Source: three-view drawing plus pictorial views. Frame: mm from the lowest corner of the part. Give positions to 0.01 mm unless a question says otherwise; leave off trailing zeros. Loops run counter-clockwise (first coordinate to the right, second up) from the corner with the lowest first, then second, coordinate; pieces in that order, holes last. Notation, with made-up numbers: M 28.5,68.25 L 32.5,68.25 A19 cw 32.5,85.25 Z; hole C 76.25,85.5 d7. An arc over 180 degrees is marked long. One line per item, written item: value. Start each with the question number.
(1) Ray query, line 1 along Y through (x, z) = (39.95, 2.3); line 2 along Y through (x, z) = (27.5, 2.1); line 3 along X through (y, z) = (59, 1.25). Return the intervals inside material, ascending. Write a range as from..to.
(2) Section B-B on x = 27.5. Output: boundary loops of the cut face in (y, z).
(3) Pin query (flat end, axial travel): P1, Ø1, axis at x = 29.5, z = 1.5, coming from the -Y side; P2, Ø1.9, axis at x = 27.5, y = 55.05, coming from the -Z side. Return the tip coordinate at first contact, or that it passes through.
(4) Section C-C on z = 0.75. Output: boundary loops of the cut face in (x, y).
(5) Section A-A on y = 55.05. Output: boundary loops of the cut face in (x, z).
(6) Section D-D on y = 17.55. Output: boundary loops of the cut face in (x, z).
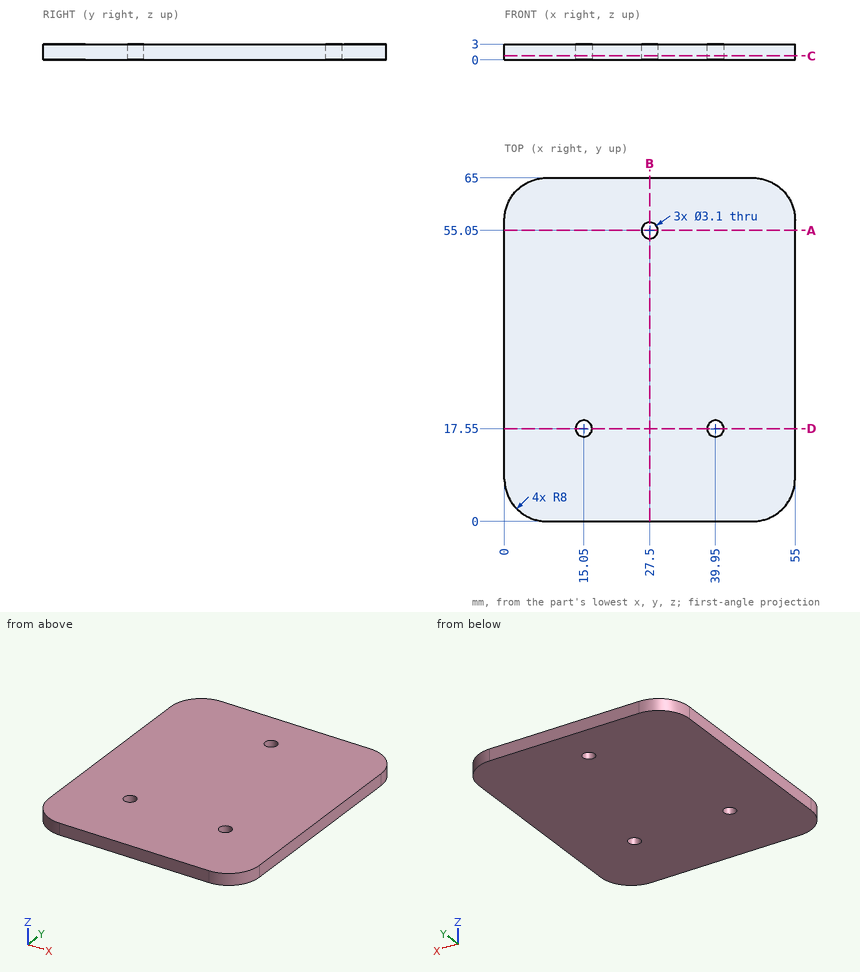
Output values:
1. line 1: y = 0..16, 19.1..65
1. line 2: y = 0..53.5, 56.6..65
1. line 3: x = 0.25..54.75
2. outline: M 0,0 L 53.5,0 L 53.5,3 L 0,3 Z; M 56.6,0 L 65,0 L 65,3 L 56.6,3 Z
3. P1: stops at y = 0
3. P2: passes through
4. outline: M 0,8 A8 ccw 8,0 L 47,0 A8 ccw 55,8 L 55,57 A8 ccw 47,65 L 8,65 A8 ccw 0,57 Z; hole C 15.05,17.55 d3.1; hole C 27.5,55.05 d3.1; hole C 39.95,17.55 d3.1
5. outline: M 0,0 L 25.95,0 L 25.95,3 L 0,3 Z; M 29.05,0 L 55,0 L 55,3 L 29.05,3 Z
6. outline: M 0,0 L 13.5,0 L 13.5,3 L 0,3 Z; M 16.6,0 L 38.4,0 L 38.4,3 L 16.6,3 Z; M 41.5,0 L 55,0 L 55,3 L 41.5,3 Z
